```python
from build123d import *

# Parameters (mm, degrees)
BOSS_EXTRUDE1_DEPTH   = 12.7
BOSS_EXTRUDE1_2_DEPTH = 12.7
BOSS_EXTRUDE1_3_DEPTH = 12.7
SKETCH3_R             = 35.68082971
BOSS_EXTRUDE2_DEPTH   = 1
CUT_EXTRUDE1_DEPTH    = 3
BOSS_EXTRUDE3_START   = 7
BOSS_EXTRUDE3_DEPTH   = 7


with BuildPart() as part:
    # Sketch2 → Boss-Extrude1 (new body)
    with BuildSketch(Plane.XY):
        with BuildLine():
            Line((-39.100035207, -47.596183278), (-14.633983159, -52.182948751))
            ThreePointArc((-14.633983159, -52.182948751), (-13.835344136, -43.767548454), (-15.038788838, -35.400439796))
            Line((-15.038788838, -35.400439796), (-39.255245143, -41.161460912))
            ThreePointArc((-39.255245143, -41.161460912), (-38.688115422, -44.36701442), (-39.100035207, -47.596183278))
        make_face()
    extrude(amount=BOSS_EXTRUDE1_DEPTH)



with BuildPart() as body_2:
    # Sketch2 → Boss-Extrude1 2 (new body)
    with BuildSketch(Plane.XY):
        with BuildLine():
            Line((-52.138110144, -34.132169435), (-60.398880747, -10.650564096))
            ThreePointArc((-60.398880747, -10.650564096), (-68.086150698, -14.166622561), (-74.730557001, -19.392390574))
            Line((-74.730557001, -19.392390574), (-57.633138211, -37.483946366))
            ThreePointArc((-57.633138211, -37.483946366), (-55.1406123, -35.390020866), (-52.138110144, -34.132169435))
        make_face()
    extrude(amount=BOSS_EXTRUDE1_2_DEPTH)


with BuildPart() as body_3:
    # Sketch2 → Boss-Extrude1 3 (new body)
    with BuildSketch(Plane.XY):
        with BuildLine():
            Line((-58.748050211, -79.091002811), (-51.629012696, -55.238425903))
            ThreePointArc((-51.629012696, -55.238425903), (-54.688668329, -54.126797895), (-57.2792507, -52.155480469))
            Line((-57.2792507, -52.155480469), (-73.484532144, -71.050320335))
            ThreePointArc((-73.484532144, -71.050320335), (-66.595901216, -75.949662166), (-58.748050211, -79.091002811))
        make_face()
    extrude(amount=BOSS_EXTRUDE1_3_DEPTH)


with BuildPart() as part_1:
    add(part.part)

    add(body_2.part)  # Boss-Extrude2 merges body 2
    # Sketch3 → Boss-Extrude2 (add)
    with BuildSketch(Plane.XY.offset(12.7)):
        with Locations(Location((-49.505798683, -44.627944394, 0), (0, 0, 134.987742115))):
            Circle(SKETCH3_R)
    extrude(amount=BOSS_EXTRUDE2_DEPTH)


with BuildPart() as cut_extrude1_tool:
    # Sketch4 → Cut-Extrude1 (new body)
    with BuildSketch(Plane(origin=(0, 0, 0), x_dir=(-1, 0, 0), z_dir=(0, 0, -1))):
        with BuildLine():
            Line((72.786303474, -71.004238215), (57.24818113, -52.887284523))
            ThreePointArc((57.24818113, -52.887284523), (54.928154107, -54.565713106), (52.261209215, -55.608331369))
            Line((52.261209215, -55.608331369), (59.087161374, -78.478915843))
            ThreePointArc((59.087161374, -78.478915843), (66.356415438, -75.510746955), (72.786303474, -71.004238215))
        make_face()
        with BuildLine():
            Line((38.618799354, -41.524006424), (15.39931612, -36.000162163))
            ThreePointArc((15.39931612, -36.000162163), (14.335198748, -43.779605292), (15.023005781, -51.601306045))
            Line((15.023005781, -51.601306045), (38.48180909, -47.203374214))
            ThreePointArc((38.48180909, -47.203374214), (38.18826081, -44.354957583), (38.618799354, -41.524006424))
        make_face()
        with BuildLine():
            Line((57.637387481, -36.751495388), (74.030918556, -19.404755176))
            ThreePointArc((74.030918556, -19.404755176), (67.825781865, -14.593480934), (60.708086795, -11.278288922))
            Line((60.708086795, -11.278288922), (52.78740583, -33.793174445))
            ThreePointArc((52.78740583, -33.793174445), (55.400981133, -34.963162493), (57.637387481, -36.751495388))
        make_face()
    extrude(amount=-CUT_EXTRUDE1_DEPTH)


with BuildPart() as part_2:
    add(part_1.part)

    # Cut-Extrude1: cut by cut_extrude1_tool
    add(cut_extrude1_tool.part, mode=Mode.SUBTRACT)



with BuildPart() as body_3_1:
    add(body_3.part)

    # Cut-Extrude1: cut by cut_extrude1_tool
    add(cut_extrude1_tool.part, mode=Mode.SUBTRACT)


with BuildPart() as part_3:
    add(part_2.part)

    add(body_3_1.part)  # Boss-Extrude3 merges body 3
    # Sketch5 → Boss-Extrude3 (add)
    with BuildSketch(Plane(origin=(0, 0, 12.7), x_dir=(-1, 0, 0), z_dir=(0, 0, -1)).offset(BOSS_EXTRUDE3_START)):
        with BuildLine():
            Line((73.484532144, -71.050320335), (73.148515106, -70.680060224))
            ThreePointArc((73.148515106, -70.680060224), (84.676398619, -45.476283496), (74.377079258, -19.746019596))
            Line((74.377079258, -19.746019596), (74.730557001, -19.392390574))
            ThreePointArc((74.730557001, -19.392390574), (85.176253231, -45.488340334), (73.484532144, -71.050320335))
        make_face()
        with BuildLine():
            Line((14.633983159, -52.182948751), (15.122646341, -52.077079515))
            ThreePointArc((15.122646341, -52.077079515), (31.185815502, -74.662407853), (58.618537366, -78.608067595))
            Line((58.618537366, -78.608067595), (58.748050211, -79.091002811))
            ThreePointArc((58.748050211, -79.091002811), (30.925446669, -75.089266226), (14.633983159, -52.182948751))
        make_face()
        with BuildLine():
            Line((15.521779426, -35.529745991), (15.038788838, -35.400439796))
            ThreePointArc((15.038788838, -35.400439796), (32.415696151, -13.306226622), (60.398880747, -10.650564096))
            Line((60.398880747, -10.650564096), (60.246234604, -11.126693443))
            ThreePointArc((60.246234604, -11.126693443), (32.655181929, -13.745141832), (15.521779426, -35.529745991))
        make_face()
    extrude(amount=-BOSS_EXTRUDE3_DEPTH)


solid = part_3.part
```
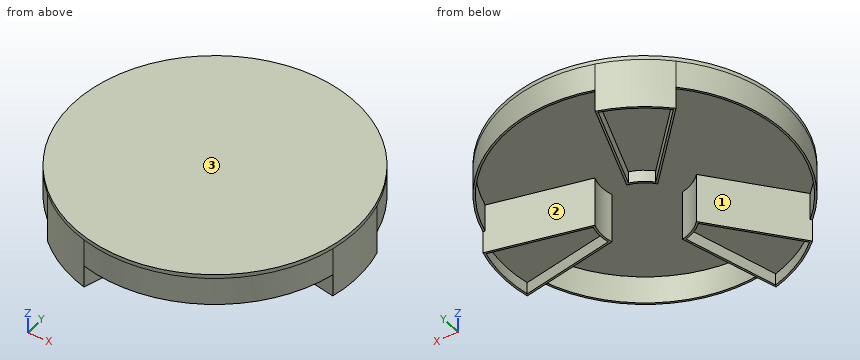
The listing builds one solid part. Answer for the finished solid, in the listing's coordinates (mm). Face numbers are marked on the shaded views. Give positions to 0.01 mm unless a question says otherwise; leave off trailing zeros. Order: outer loops, then holes, each group sorted by start corner. A loop starts at its lowest first (then second) coordinate and runs counter-clockwise, first axis right, second up.
1) Given P1, Ø8, axis at x = -22, y = -47, coming from the -Z side; P2, Ø6, axis at y = -68, z = 10, coming from the +X side; P3, Ø22.5, axis at x = -40.5, y = -64.5, coming from the -Z side; P4, Ø8, axis at y = -59.5, z = 6.5, coming from the +X side, each flat-ended and moving along its own axis, determine where each tip first touches the part or whether it passes through.
Reported:
P1: stops at z = 0
P2: stops at x = -20.21
P3: stops at z = 12.7
P4: stops at x = -15.52
2) Find section D-D on y = -24.5. Write down the section's boundary in (x, z).
Reported:
outline: (-78.97, 5.7) - (-78.36, 5.7) - (-78.36, 12.7) - (-69.9, 12.7) - (-69.9, 0) - (-69.22, 0) - (-69.22, 3) - (-56.06, 3) - (-56.06, 0) - (-55.53, 0) - (-55.53, 12.7) - (-20.65, 12.7) - (-20.65, 5.7) - (-20.04, 5.7) - (-20.04, 13.7) - (-78.97, 13.7) - close
3) Find section B-B on z = 6.75. Write down the section's boundary in (x, y) (3 decimals), then the cut area to 3 significant figures.
Reported:
outline: circle Ø71.362 at (-49.506, -44.628); hole (-74.387, -19.756) arc R35.181 ccw to (-73.159, -70.671) - (-57.279, -52.155) arc R10.821 ccw to (-51.629, -55.238) - (-58.605, -78.612) arc R35.181 ccw to (-15.126, -52.091) - (-39.1, -47.596) arc R10.821 ccw to (-39.255, -41.161) - (-15.525, -35.516) arc R35.181 ccw to (-60.233, -11.122) - (-52.138, -34.132) arc R10.821 ccw to (-57.633, -37.484) - close
area: 962 mm2
4) Consider line 1 along X through (y, z) = (-53, 11); line 2 along X through (y, z) = (-45, 9.5); line 3 along X through (y, z) = (-54, 12.25). Determine where each line is inside the solid, lowest interval first.
Reported:
line 1: x = -84.19 to -83.68, -58 to -56.36, -15.34 to -14.82
line 2: x = -85.18 to -84.68, -38.69 to -13.83
line 3: x = -83.93 to -83.42, -58.86 to -54.91, -15.6 to -15.08
5) Determine the mould class of the marked faces 1, 2 and 3 for opening direction Y: pulls with the +Y half, pulls with the -Y half, needs draft (parallel to the pull), parting line crosses it, or undercut.
Reported:
face 1: undercut
face 2: undercut
face 3: needs draft
6) Find section A-A on z = 1.75. Write down the section's boundary in (x, y), then the cut area to 3 significant figures.
Reported:
outline: (-74.73, -19.39) - (-57.63, -37.48) arc R10.82 cw to (-52.14, -34.13) - (-60.4, -10.65) arc R35.68 ccw to start; (-73.48, -71.05) arc R35.68 ccw to (-58.75, -79.09) - (-51.63, -55.24) arc R10.82 cw to (-57.28, -52.16) - close; (-39.26, -41.16) arc R10.82 cw to (-39.1, -47.6) - (-14.63, -52.18) arc R35.68 ccw to (-15.04, -35.4) - close; hole (-74.03, -19.4) - (-57.64, -36.75) arc R11.32 cw to (-52.79, -33.79) - (-60.71, -11.28) arc R35.18 ccw to start; hole (-72.79, -71) arc R35.18 ccw to (-59.09, -78.48) - (-52.26, -55.61) arc R11.32 cw to (-57.25, -52.89) - close; hole (-38.62, -41.52) arc R11.32 cw to (-38.48, -47.2) - (-15.02, -51.6) arc R35.18 ccw to (-15.4, -36) - close
area: 107 mm2
7) Find section C-C on x = -21. Write down the section's boundary in (y, z).
Reported:
outline: (-66.09, 5.7) - (-65.25, 5.7) - (-65.25, 12.7) - (-50.99, 12.7) - (-50.99, 0) - (-50.48, 0) - (-50.48, 3) - (-37.33, 3) - (-37.33, 0) - (-36.82, 0) - (-36.82, 12.7) - (-24.01, 12.7) - (-24.01, 5.7) - (-23.17, 5.7) - (-23.17, 13.7) - (-66.09, 13.7) - close
